from build123d import *

# Parameters (mm, degrees)
BOSS_EXTRU_1_DEPTH      = 10
ESQUISSE2_R             = 2.1
BOSS_EXTRU_2_DEPTH      = 45
ENL_V_MAT_EXTRU_1_DEPTH = 2.5
CONG_1_R                = 5


with BuildPart() as part:
    # Esquisse1 → Boss.-Extru.1 (new body)
    with BuildSketch(Plane.XY):
        Polygon((16.90473047, -36.252311481), (26.618508055, -31.722702604), (38.913655488, -14.163412304), (40.781920359, 7.190952884), (31.722702604, 26.618508055), (-26.618508055, 31.722702604), (-38.913655488, 14.163412304), (-40.781920359, -7.190952884), (-31.722702604, -26.618508055), (-22.943057454, -32.766081772), align=None)
    extrude(amount=BOSS_EXTRU_1_DEPTH)

    # Esquisse2 → Boss.-Extru.2 (add)
    with BuildSketch(Plane.XY.offset(10)):
        Polygon((31.722702604, 26.618508055), (-26.618508055, 31.722702604), (-38.913655488, 14.163412304), (-40.781920359, -7.190952884), (-31.722702604, -26.618508055), (-22.943057454, -32.766081772), (16.90473047, -36.252311481), (26.618508055, -31.722702604), (38.913655488, -14.163412304), (40.781920359, 7.190952884), align=None)
        with Locations(Location((34.806654387, -3.73808347, 0), (0, 0, 180))):
            Circle(ESQUISSE2_R, mode=Mode.SUBTRACT)
        with Locations(Location((29.737818366, -18.469938184, 0), (0, 0, 180))):
            Circle(ESQUISSE2_R, mode=Mode.SUBTRACT)
        with Locations(Location((-32.981605632, -11.73414452, 0), (0, 0, 180))):
            Circle(ESQUISSE2_R, mode=Mode.SUBTRACT)
        with Locations(Location((-34.806654387, 3.73808347, 0), (0, 0, 180))):
            Circle(ESQUISSE2_R, mode=Mode.SUBTRACT)
        with Locations(Location((-29.737818366, 18.469938184, 0), (0, 0, 180))):
            Circle(ESQUISSE2_R, mode=Mode.SUBTRACT)
        with Locations(Location((32.981605632, 11.73414452, 0), (0, 0, 180))):
            Circle(ESQUISSE2_R, mode=Mode.SUBTRACT)
        with Locations(Location((18.601253659, -30.822032576, 0), (0, 0, 180))):
            Circle(ESQUISSE2_R, mode=Mode.SUBTRACT)
        with Locations(Location((-22.943057454, -28.537832938, 0), (0, 0, 180))):
            Circle(ESQUISSE2_R, mode=Mode.SUBTRACT)
        with Locations(Location((26.618508055, 22.705871893, 0), (0, 0, 180))):
            Circle(ESQUISSE2_R, mode=Mode.SUBTRACT)
        with Locations(Location((-22.943057454, 26.554275329, 0), (0, 0, 180))):
            Circle(ESQUISSE2_R, mode=Mode.SUBTRACT)
        Polygon((-20.194060765, 21.161060665), (-29.41542134, 7.991592941), (-30.816619994, -8.024180951), (-24.022206677, -22.594847329), (-10.852738952, -31.816207904), (5.163034939, -33.217406557), (19.733701317, -26.42299324), (28.955061892, -13.253525516), (30.356260545, 2.762248376), (23.561847229, 17.332914754), (10.392379504, 26.554275329), (-5.623394388, 27.955473982), align=None, mode=Mode.SUBTRACT)
    extrude(amount=BOSS_EXTRU_2_DEPTH)

    # Esquisse3 → Enlèv. mat.-Extru.1 (cut)
    with BuildSketch(Plane.XY.offset(55)):
        Polygon((-34.806654387, -0.37842395), (-31.241654387, 1.67982976), (-31.241654387, 5.796337179), (-34.806654387, 7.854590889), (-38.371654387, 5.796337179), (-38.371654387, 1.67982976), align=None)
        Polygon((-22.943057454, 22.426220904), (-19.368057454, 24.490248116), (-19.368057454, 28.618302541), (-22.943057454, 30.682329753), (-26.518057454, 28.618302541), (-26.518057454, 24.490248116), align=None)
        Polygon((30.193508055, 20.641844681), (30.193508055, 24.769899106), (26.618508055, 26.833926318), (23.043508055, 24.769899106), (23.043508055, 20.641844681), (26.618508055, 18.577817469), align=None)
        Polygon((38.381654387, -5.802110682), (38.381654387, -1.674056257), (34.806654387, 0.389970955), (31.231654387, -1.674056257), (31.231654387, -5.802110682), (34.806654387, -7.866137894), align=None)
    extrude(amount=-ENL_V_MAT_EXTRU_1_DEPTH, mode=Mode.SUBTRACT)

    # Congé1
    cong_1_edges = [part.edges().sort_by_distance(p)[0] for p in [
        (40.781920359, 7.190952884, 27.5),
        (38.913655488, -14.163412304, 27.5),
        (26.618508055, -31.722702604, 27.5),
        (-31.722702604, -26.618508055, 27.5),
        (-40.781920359, -7.190952884, 27.5),
        (-38.913655488, 14.163412304, 27.5),
    ]]
    fillet(cong_1_edges, radius=CONG_1_R)


solid = part.part
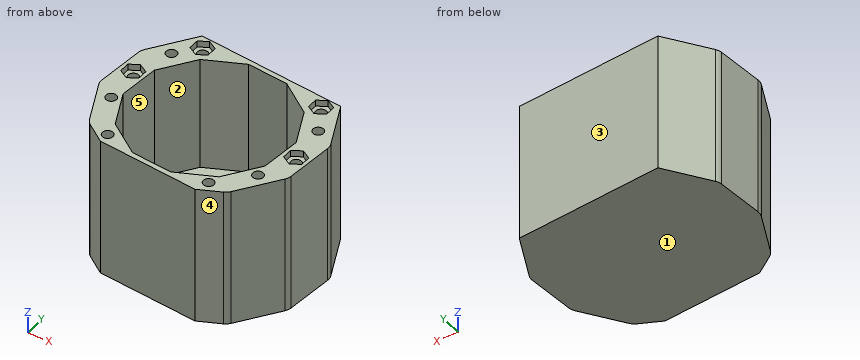
The listing builds one solid part. Answer for the finished solid, in the listing's coordinates (mm). Face numbers are marked on the shaded views. A direction names the side the tool comes from. Coordinates: 2 decimals unless noted, no trailing zeros. Write each loop counter-clockwise with the first axis right and the second up, starting at its lowest first coordinate (ties: lowest second). Pieces come first, ordered by that corner, then holes. Notation, with made-up numbers: M -11,69 L 1,69 A25 cw 1,91 Z; hole C -15,40 d5. An arc over 180 degrees is marked long. Use one line per item in the form item = value.
Item 1: Find the intervals of material crossed by probe 1 along X at (y, z) = (5, 53.5); probe 2 along X at (y, z) = (18, 34.5); probe 3 along X at (y, z) = (-29.5, 50), in increasing order.
Model answer:
probe_1 = -39.72 to -38.37, -31.24 to -29.68, 29.31 to 40.59
probe_2 = -36.23 to -31.78, -27.69 to -22.41, 22.61 to 35.74
probe_3 = -27.61 to -24.81, -21.08 to -14.16, 13.14 to 16.97, 20.23 to 28.17
Item 2: Given P1, Ø2, axis at y = 21.5, z = 54, coming from the -X side; P2, Ø8, axis at x = -1, y = -1.5, coming from the +Z side; P3, Ø5, axis at x = -5.5, z = 8.5, coming from the -Y side; P4, Ø6.5, axis at x = 32.98, y = 11.73, coming from the -Z side, each flat-ended and moving along its own axis, determine where each tip first touches the part or whether it passes through.
Model answer:
P1 = -34.48
P2 = 10
P3 = -34.51
P4 = 0
Item 3: Find section A-A, the plane z = 7. Give the vertices of the cut face in (x, y), plus the area to 3 significant figures.
Model answer:
outline = M -40.67,-5.86 A5 ccw -40.22,-8.41 L -32.29,-25.4 A5 ccw -30.63,-27.39 L -22.94,-32.77 L 16.9,-36.25 L 25.4,-32.29 A5 ccw 27.39,-30.63 L 38.15,-15.26 A5 ccw 39.03,-12.83 L 40.67,5.86 A5 ccw 40.22,8.41 L 31.72,26.62 L -26.62,31.72 L -38.15,15.26 A5 ccw -39.03,12.83 Z
area = 4,550 mm2
Item 4: Find section C-C, the plane z = 22. Give the number of separate pieces and of enclosed holes in the cut face, plus the area to 3 significant figures.
Model answer:
separate_pieces = 1
enclosed_holes = 11
area = 1,520 mm2
Item 5: For the marked faces 4 and 5, determine the directions among +Z, -Z, +X, -X, +Y, -Y from which every point of the face is accessible in a straight line to the end or side of a thin tool.
Model answer:
face_4 = +Z, -Z, +X, -Y
face_5 = +Z
Item 6: Find section B-B, the plane x = 13. Give the vertices of the cut face in (y, z).
Model answer:
outline = M -35.91,0 L 28.26,0 L 28.26,55 L 24.73,55 L 24.73,10 L -29.56,10 L -29.56,55 L -35.91,55 Z
Item 7: Find section D-D, the plane x = -0.5. Give the vertices of the cut face in (y, z), plus the area to 3 significant figures.
Model answer:
outline = M -34.73,0 L 29.44,0 L 29.44,55 L 27.51,55 L 27.51,10 L -32.72,10 L -32.72,55 L -34.73,55 Z
area = 819 mm2
Item 8: The mould has two halves that part along Y. Classify the marked faces 1, 2 and 3: released by +Y, released by -Y, zero draft, split by the parting line, or undercut.
Model answer:
face_1 = zero draft
face_2 = undercut
face_3 = released by +Y
